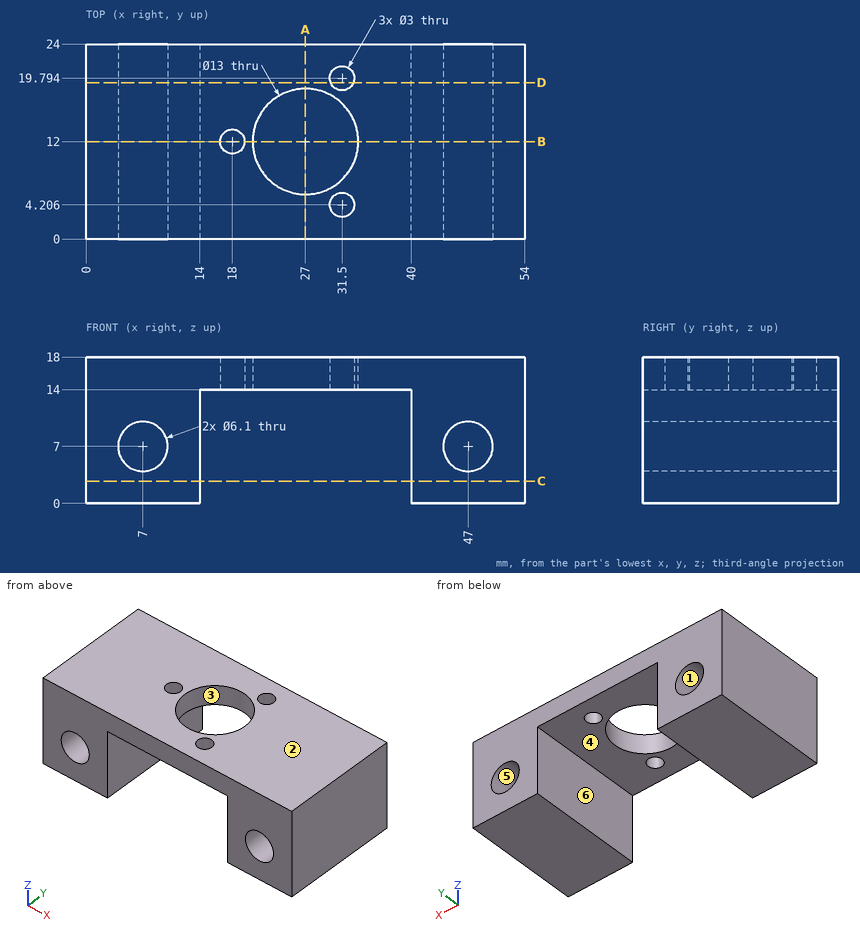
Drawing for the job (mm, zero at the part's lowest x, y, z). A direction names the side the tool comes from. Give positions to 0.01 mm unless a question says otherwise; leave off trailing zeros. Write each loop counter-clockwise with the first axis right and the second up, starting at its lowest first coordinate (ties: lowest second). Pieces come first, ordered by that corner, then holes. Notation, with made-up numbers: M -5.75,42.25 L 21.25,42.25 A26 cw 21.25,65.25 Z; hole C 85,0 d7. An arc over 180 degrees is marked long. Return JSON: item names as keys, results as strings. Group by question number.
(1) 3-axis set-ups, long thin cutter, end or side, ignore diameter. For the marked faces 5 and 6: which of +Z, -Z, +X, -X, +Y, -Y reach the whole face in a straight line?
(2) Band-saw the part on B-B (y = 12). Give the cut face in (x, z).
(3) Band-saw the part on A-A (x = 27). Give the cut face in (y, z), and give its area (3 significant figures).
(4) Flat gauge pins, fed straight in: pin 1 Ø4 at (x, y) = (18, 12) entering from +Z; pin 2 Ø3.5 at (x, y) = (31.5, 4.21) entering from -Z. Where does each tip first touch, or does it go through?
(5) Drill centre lines: L1, parallel to X at y = 5.5, z = 7; L2, parallel to X at y = 1.5, z = 13; L3, parallel to X at y = 15, z = 4.75. Where is each one in solid material? Low to high. Write a range as [from, to].
(6) Band-saw the part on C-C (z = 2.75). Give the cut face in (x, y), and give its area (3 significant figures).
(7) Band-saw the part on D-D (y = 19.25). Give the cut face in (x, z), and give its area (3 significant figures).
(8) Mould opens along Z. For the marked faces 1, 2, 3 and 4 say: pulls with the +Z half, pulls with the -Z half, needs draft (parallel to the pull), parting line crosses it, or undercut.
Entries:
{
 "1": {"face 5": "+Y, -Y", "face 6": "-Z, +Y, -Y"},
 "2": {"outline": "M 0,0 L 14,0 L 14,14 L 16.5,14 L 16.5,18 L 0,18 Z; M 19.5,14 L 20.5,14 L 20.5,18 L 19.5,18 Z; M 33.5,14 L 40,14 L 40,0 L 54,0 L 54,18 L 33.5,18 Z; hole C 7,7 d6.1; hole C 47,7 d6.1"},
 "3": {"outline": "M 0,14 L 5.5,14 L 5.5,18 L 0,18 Z; M 18.5,14 L 24,14 L 24,18 L 18.5,18 Z", "area": "44.0 mm^2"},
 "4": {"pin 1": "stops at z = 18", "pin 2": "stops at z = 14"},
 "5": {"L1": "x = [0, 3.95], [10.05, 14], [40, 43.95], [50.05, 54]", "L2": "x = [0, 14], [40, 54]", "L3": "x = [0, 4.94], [9.06, 14], [40, 44.94], [49.06, 54]"},
 "6": {"outline": "M 0,0 L 14,0 L 14,24 L 0,24 Z; M 40,0 L 54,0 L 54,24 L 40,24 Z", "area": "672 mm^2"},
 "7": {"outline": "M 0,0 L 14,0 L 14,14 L 30.1,14 L 30.1,18 L 0,18 Z; M 32.9,14 L 40,14 L 40,0 L 54,0 L 54,18 L 32.9,18 Z; hole C 7,7 d6.1; hole C 47,7 d6.1", "area": "538 mm^2"},
 "8": {"face 1": "undercut", "face 2": "pulls with the +Z half", "face 3": "needs draft", "face 4": "pulls with the -Z half"}
}
